Geometry: final body of the model. Coordinates: model frame, mm. Face numbers are marked on the shaded views. Give positions to 0.01 mm unless a question says otherwise; leave off trailing zeros. Write each loop counter-clockwise with the first axis right and the second up, starting at its lowest first coordinate (ties: lowest second). Pieces come first, ordered by that corner, then holes.
from build123d import *

# Parameters (mm, degrees)
ESQUISSE1_R             = 1.25
BOSS_EXTRU_1_DEPTH      = 8
ESQUISSE5_W             = 45.3176151
ESQUISSE5_H             = 84.101601091
ESQUISSE5_R             = 2.5
ENL_V_MAT_EXTRU_2_DEPTH = 3
ESQUISSE6_W             = 5
ESQUISSE6_H             = 62
BOSS_DC_DC_DEPTH        = 2
ENL_V_INDUCTORS_DEPTH   = 2
ESQUISSE8_W             = 154.760825025
ESQUISSE8_H             = 103.254487946
ENL_V_MAT_EXTRU_3_DEPTH = 0.5


with BuildPart() as part:
    # Esquisse1 → Boss.-Extru.1 (new body)
    with BuildSketch(Plane.XY):
        with BuildLine():
            Line((43.290045774, 103.030192742), (43.290045774, 179.130192742))
            ThreePointArc((43.290045774, 179.130192742), (44.16872543, 181.251513085), (46.290045774, 182.130192742))
            Line((46.290045774, 182.130192742), (75.290045774, 182.130192742))
            ThreePointArc((75.290045774, 182.130192742), (77.411366118, 181.251513085), (78.290045774, 179.130192742))
            Line((78.290045774, 179.130192742), (78.290045774, 103.030192742))
            ThreePointArc((78.290045774, 103.030192742), (79.16872543, 100.908872398), (81.290045774, 100.030192742))
            Line((81.290045774, 100.030192742), (146.96841177, 100.030192742))
            ThreePointArc((146.96841177, 100.030192742), (149.089732114, 99.151513085), (149.96841177, 97.030192742))
            Line((149.96841177, 97.030192742), (149.96841177, 3.030192742))
            ThreePointArc((149.96841177, 3.030192742), (149.089732114, 0.908872398), (146.96841177, 0.030192742))
            Line((146.96841177, 0.030192742), (2.96841177, 0.030192742))
            ThreePointArc((2.96841177, 0.030192742), (0.847091427, 0.908872398), (-0.03158823, 3.030192742))
            Line((-0.03158823, 3.030192742), (-0.03158823, 97.030192742))
            ThreePointArc((-0.03158823, 97.030192742), (0.847091427, 99.151513085), (2.96841177, 100.030192742))
            Line((2.96841177, 100.030192742), (40.290045774, 100.030192742))
            ThreePointArc((40.290045774, 100.030192742), (42.411366118, 100.908872398), (43.290045774, 103.030192742))
        make_face()
        with Locations((12.96841177, 92.530192742)):
            Circle(ESQUISSE1_R, mode=Mode.SUBTRACT)
        with Locations((74.96841177, 92.530192742)):
            Circle(ESQUISSE1_R, mode=Mode.SUBTRACT)
        with Locations((136.96841177, 92.530192742)):
            Circle(ESQUISSE1_R, mode=Mode.SUBTRACT)
        with Locations((12.96841177, 50.030192742)):
            Circle(ESQUISSE1_R, mode=Mode.SUBTRACT)
        with Locations((74.96841177, 50.030192742)):
            Circle(ESQUISSE1_R, mode=Mode.SUBTRACT)
        with Locations((136.96841177, 50.030192742)):
            Circle(ESQUISSE1_R, mode=Mode.SUBTRACT)
        with Locations((136.96841177, 7.530192742)):
            Circle(ESQUISSE1_R, mode=Mode.SUBTRACT)
        with Locations((74.96841177, 7.530192742)):
            Circle(ESQUISSE1_R, mode=Mode.SUBTRACT)
        with Locations((12.96841177, 7.530192742)):
            Circle(ESQUISSE1_R, mode=Mode.SUBTRACT)
        with Locations((46.790045774, 178.530192742)):
            Circle(ESQUISSE1_R, mode=Mode.SUBTRACT)
        with Locations((74.790045774, 178.530192742)):
            Circle(ESQUISSE1_R, mode=Mode.SUBTRACT)
    extrude(amount=BOSS_EXTRU_1_DEPTH)

    # Esquisse5 → Enlèv. mat.-Extru.2 (cut)
    with BuildSketch(Plane(origin=(0, 0, 0), x_dir=(-1, 0, 0), z_dir=(0, 0, -1))):
        with Locations((-61.04710063, 142.080993288)):
            Rectangle(ESQUISSE5_W, ESQUISSE5_H)
        with Locations((-74.790045774, 178.530192742)):
            Circle(ESQUISSE5_R, mode=Mode.SUBTRACT)
        with Locations((-46.790045774, 178.530192742)):
            Circle(ESQUISSE5_R, mode=Mode.SUBTRACT)
    extrude(amount=-ENL_V_MAT_EXTRU_2_DEPTH, mode=Mode.SUBTRACT)

    # Esquisse6 → Boss.-DC/DC (add)
    with BuildSketch(Plane(origin=(0, 0, 3), x_dir=(-1, 0, 0), z_dir=(0, 0, -1))):
        with Locations((-53.290045774, 134.530192742)):
            Rectangle(ESQUISSE6_W, ESQUISSE6_H)
    extrude(amount=BOSS_DC_DC_DEPTH)

    # Esquisse7 → Enlèv. Inductors (cut)
    with BuildSketch(Plane(origin=(0, 0, 3), x_dir=(-1, 0, 0), z_dir=(0, 0, -1))):
        with BuildLine():
            Line((-73.790045774, 167.530192742), (-65.790045774, 167.530192742))
            ThreePointArc((-65.790045774, 167.530192742), (-64.375832212, 166.944406304), (-63.790045774, 165.530192742))
            Line((-63.790045774, 165.530192742), (-63.790045774, 107.530192742))
            ThreePointArc((-63.790045774, 107.530192742), (-64.375832212, 106.115979179), (-65.790045774, 105.530192742))
            Line((-65.790045774, 105.530192742), (-73.790045774, 105.530192742))
            ThreePointArc((-73.790045774, 105.530192742), (-75.204259336, 106.115979179), (-75.790045774, 107.530192742))
            Line((-75.790045774, 107.530192742), (-75.790045774, 165.530192742))
            ThreePointArc((-75.790045774, 165.530192742), (-75.204259336, 166.944406304), (-73.790045774, 167.530192742))
        make_face()
    extrude(amount=-ENL_V_INDUCTORS_DEPTH, mode=Mode.SUBTRACT)

    # Esquisse8 → Enlèv. mat.-Extru.3 (cut)
    with BuildSketch(Plane(origin=(0, 0, 0), x_dir=(-1, 0, 0), z_dir=(0, 0, -1))):
        with Locations((-74.96841177, 50.092755489)):
            Rectangle(ESQUISSE8_W, ESQUISSE8_H)
    extrude(amount=-ENL_V_MAT_EXTRU_3_DEPTH, mode=Mode.SUBTRACT)


solid = part.part
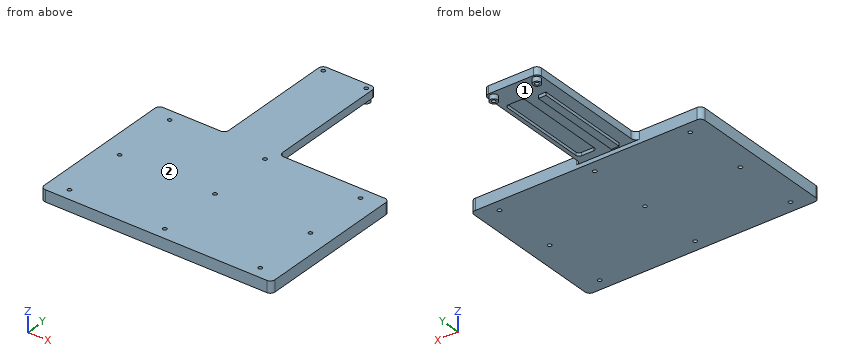
Q1. Section D-D on x = 96. Output: boundary loops of the cut face in (y, z), plus the area to 3 significant figures.
Filled sheet:
outline: (0.03, 0.5) - (100.03, 0.5) - (100.03, 8) - (0.03, 8) - close
area: 750 mm2
Q2. Pull-direction query (Y, two-part tool) for the marked faces 1 and 2; classes: released by +Y, released by -Y, zero draft, split by the parting line, or undercut.
Filled sheet:
face 1: undercut
face 2: zero draft
Q3. Pin query (flat end, axial travel): P1, Ø1, axis at x = 123.5, y = 40.5, coming from the -Z side; P2, Ø2, axis at x = 83, z = 4, coming from the +Y side; P3, Ø20.5, axis at x = 56.5, y = 126.5, coming from the -Z side. Return the tip coordinate at first contact, or that it passes through.
Filled sheet:
P1: stops at z = 0.5
P2: stops at y = 100.03
P3: stops at z = 1
Q4. Ray query, line 1 along Y through (x, z) = (143.5, 3.25); line 2 along Z through (x, y) = (42.5, 89); line 3 along Y through (x, z) = (74.5, 2.5). Return the intervals inside material, ascending.
Filled sheet:
line 1: y = 0.03 to 100.03
line 2: z = 0.5 to 8
line 3: y = 0.03 to 6.37, 8.69 to 48.87, 51.19 to 91.37, 93.69 to 100.03, 176.05 to 177.31, 179.75 to 181.01
Q5. Section A-A on x = 68. Output: boundary loops of the cut face in (y, z), plus the area to 3 significant figures.
Filled sheet:
outline: (0.03, 0.5) - (100.03, 0.5) - (100.03, 3) - (105.53, 3) - (105.53, 5) - (167.53, 5) - (167.53, 3) - (182.13, 3) - (182.13, 8) - (0.03, 8) - close
area: 1,040 mm2
Q6. Section C-C on y = 158. Output: boundary loops of the cut face in (x, z), plus the area to 3 significant figures.
Filled sheet:
outline: (43.29, 3) - (50.79, 3) - (50.79, 1) - (55.79, 1) - (55.79, 3) - (63.79, 3) - (63.79, 5) - (75.79, 5) - (75.79, 3) - (78.29, 3) - (78.29, 8) - (43.29, 8) - close
area: 161 mm2
Q7. Section B-B on z = 6.5. Count the separate pieces of the cut face and the enclosed holes in it, plus the area to 3 significant figures.
Filled sheet:
separate pieces: 1
enclosed holes: 11
area: 17,800 mm2
